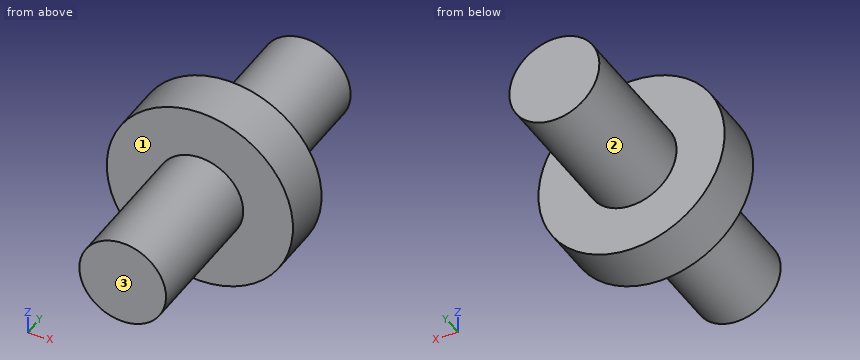
from build123d import *

# Parameters (mm, degrees)
SKETCH2_R           = 2.175
BOSS_EXTRUDE2_DEPTH = 8
SKETCH5_R           = 2.095
BOSS_EXTRUDE3_DEPTH = 8
SKETCH7_R           = 4.5
BOSS_EXTRUDE4_DEPTH = 1.25


with BuildPart() as part:
    # Sketch2 → Boss-Extrude2 (new body)
    with BuildSketch(Plane(origin=(0, 0, 0), x_dir=(1, 0, 0), z_dir=(0, 1, 0))):
        with Locations(Location((0, 0, 0), (0, 0, 270))):
            Circle(SKETCH2_R)
    extrude(amount=BOSS_EXTRUDE2_DEPTH)

    # Sketch5 → Boss-Extrude3 (add)
    with BuildSketch(Plane(origin=(0, 0, 0), x_dir=(-1, 0, 0), z_dir=(0, -1, 0))):
        with Locations(Location((0, 0, 0), (0, 0, 90))):
            Circle(SKETCH5_R)
    extrude(amount=BOSS_EXTRUDE3_DEPTH)

    # Sketch7 → Boss-Extrude4 (add, symmetric)
    with BuildSketch(Plane(origin=(0, 0, 0), x_dir=(-1, 0, 0), z_dir=(0, -1, 0))):
        with Locations(Location((0, 0, 0), (0, 0, 90))):
            Circle(SKETCH7_R)
    extrude(amount=BOSS_EXTRUDE4_DEPTH, both=True)


solid = part.part
Here's how the part is built. I have some questions about the finished solid (model axes, mm). Face numbers are marked on the shaded views. A direction names the side the tool comes from. Give positions to 0.01 mm unless a question says otherwise; leave off trailing zeros. Order: outer loops, then holes, each group sorted by start corner. A loop starts at its lowest first (then second) coordinate and runs counter-clockwise, first axis right, second up. Notation, with made-up numbers: M -12,-28 L 38,-28 A33 ccw 38,1 Z; hole C 88.5,-21 d1. An arc over 180 degrees is marked long. Answer as a JSON object with one key per item and string values. Group by question number.
1) Suppose I cut it at B-B, the plane z = 0. Write out the boundary of the cut face in (x, y) (3 decimals).
2) On a 3-axis mill with a long thin cutter (end or side, diameter ignored), from which of +Z, -Z, +X, -X, +Y, -Y can I reach the whole of each face in a straight line? I mean the marked faces 1, 2 and 3. Say none if no direction works.
3) Suppose I cut it at C-C, the plane y = 4.75. Write out the boundary of the cut face in (x, z) (3 decimals), plus the area to 3 significant figures.
4) Please list where these lines run through material, in increasing order: L1, parallel to Y at x = -1.5, z = 3.5; L2, parallel to Z at x = 0, y = -1.75 (3 decimals); L3, parallel to Z at x = 2, y = 4.5. Write a range as [from, to].
5) Suppose I cut it at D-D, the plane y = -0.75. Write out the boundary of the cut face in (x, z), plus the area to 3 significant figures.
6) Suppose I cut it at A-A, the plane x = 0. Write out the boundary of the cut face in (y, z) (3 decimals).
7) I'm going to push flat-ended pins straight in: pin 1 Ø1 at (x, y) = (-3.5, 0.5) entering from +Z; pin 2 Ø1 at (x, z) = (3, -3.5) entering from +Y; pin 3 Ø4 at (y, z) = (6, -2) entering from -X (3 decimals). Where does each tip first touch, or does it pass through?
Results found:
{
 "1": {"outline": "M -4.5,-1.25 L -2.095,-1.25 L -2.095,-8 L 2.095,-8 L 2.095,-1.25 L 4.5,-1.25 L 4.5,1.25 L 2.175,1.25 L 2.175,8 L -2.175,8 L -2.175,1.25 L -4.5,1.25 Z"},
 "2": {"face 1": "-Y", "face 2": "+Y", "face 3": "+Z, -Z, +X, -X, -Y"},
 "3": {"outline": "C 0,0 d4.35", "area": "14.9 mm²"},
 "4": {"L1": "[-1.25, 1.25]", "L2": "[-2.095, 2.095]", "L3": "[-0.85, 0.85]"},
 "5": {"outline": "C 0,0 d9", "area": "63.6 mm²"},
 "6": {"outline": "M -8,-2.095 L -1.25,-2.095 L -1.25,-4.5 L 1.25,-4.5 L 1.25,-2.175 L 8,-2.175 L 8,2.175 L 1.25,2.175 L 1.25,4.5 L -1.25,4.5 L -1.25,2.095 L -8,2.095 Z"},
 "7": {"pin 1": "z = 3.35", "pin 2": "y = 1.25", "pin 3": "x = -2.175"}
}
